```python
from build123d import *

# Parameters (mm, degrees)
SKETCH1_W                = 120
SKETCH1_H                = 120
BOSS_EXTRUDE1_DEPTH      = 115
SHELL1_T                 = -5
BOSS_EXTRUDE2_START      = -5
BOSS_EXTRUDE2_DEPTH      = 10
BOSS_EXTRUDE3_DEPTH      = 5
BOSS_EXTRUDE3_DEPTH_BACK = 5


# Read off the part's stored shape, not the designer's step: Boss-Extrude2
with BuildPart() as part:
    # Sketch1 → Boss-Extrude1 (new body)
    with BuildSketch(Plane(origin=(0, 0, 0), x_dir=(1, 0, 0), z_dir=(0, 1, 0))):
        Rectangle(SKETCH1_W, SKETCH1_H)
    extrude(amount=BOSS_EXTRUDE1_DEPTH)

    # Shell1
    shell1_openings = [part.faces().sort_by_distance(p)[0] for p in [
        (0, 115, 0),
    ]]
    offset(amount=SHELL1_T, openings=shell1_openings, kind=Kind.INTERSECTION)

    # Boss-Extrude2 outline → Boss-Extrude2 (add)
    with BuildSketch(Plane(origin=(0, 0, 0), x_dir=(0.7071067811865475, 0, 0.7071067811865477), z_dir=(-0.7071067811865477, 0, 0.7071067811865475)).offset(BOSS_EXTRUDE2_START)):
        with BuildLine():
            Line((-78.852813742, 20.605551275), (-78.852813742, 25))
            ThreePointArc((-78.852813742, 25), (-79.342915027, 25.345119301), (-79.852813742, 25.660254038))
            ThreePointArc((-79.852813742, 25.660254038), (-94.852813742, 17), (-79.852813742, 8.339745962))
            ThreePointArc((-79.852813742, 8.339745962), (-79.342915027, 8.654880699), (-78.852813742, 9))
            Line((-78.852813742, 9), (-78.852813742, 13.394448725))
            ThreePointArc((-78.852813742, 13.394448725), (-79.314922525, 12.718439436), (-79.852813742, 12.101020514))
            ThreePointArc((-79.852813742, 12.101020514), (-91.852813742, 17), (-79.852813742, 21.898979486))
            ThreePointArc((-79.852813742, 21.898979486), (-79.314922525, 21.281560564), (-78.852813742, 20.605551275))
        make_face()
        with BuildLine():
            Line((-78.852813742, 106.605551275), (-78.852813742, 111))
            ThreePointArc((-78.852813742, 111), (-79.342915027, 111.345119301), (-79.852813742, 111.660254038))
            ThreePointArc((-79.852813742, 111.660254038), (-94.852813742, 103), (-79.852813742, 94.339745962))
            ThreePointArc((-79.852813742, 94.339745962), (-79.342915027, 94.654880699), (-78.852813742, 95))
            Line((-78.852813742, 95), (-78.852813742, 99.394448725))
            ThreePointArc((-78.852813742, 99.394448725), (-79.314922525, 98.718439436), (-79.852813742, 98.101020514))
            ThreePointArc((-79.852813742, 98.101020514), (-91.852813742, 103), (-79.852813742, 107.898979486))
            ThreePointArc((-79.852813742, 107.898979486), (-79.314922525, 107.281560564), (-78.852813742, 106.605551275))
        make_face()
        with BuildLine():
            ThreePointArc((78.852813742, 95), (94.852813742, 103), (78.852813742, 111))
            Line((78.852813742, 111), (78.852813742, 106.605551275))
            ThreePointArc((78.852813742, 106.605551275), (91.852813742, 103), (78.852813742, 99.394448725))
            Line((78.852813742, 99.394448725), (78.852813742, 95))
        make_face()
        with BuildLine():
            ThreePointArc((78.852813742, 9), (94.852813742, 17), (78.852813742, 25))
            Line((78.852813742, 25), (78.852813742, 20.605551275))
            ThreePointArc((78.852813742, 20.605551275), (91.852813742, 17), (78.852813742, 13.394448725))
            Line((78.852813742, 13.394448725), (78.852813742, 9))
        make_face()
    extrude(amount=BOSS_EXTRUDE2_DEPTH)

    # Sketch3 → Boss-Extrude3 (add, two sides: drawn at the far end of the back side and taken through both)
    with BuildSketch(Plane(origin=(0, 0, 0), x_dir=(0.7071067811865475, 0, -0.7071067811865476), z_dir=(0.7071067811865476, 0, 0.7071067811865475)).offset(-BOSS_EXTRUDE3_DEPTH_BACK)):
        with BuildLine():
            Line((-78.852813742, 111), (-78.852813742, 106.605551275))
            ThreePointArc((-78.852813742, 106.605551275), (-91.852813742, 103), (-78.852813742, 99.394448725))
            Line((-78.852813742, 99.394448725), (-78.852813742, 95))
            ThreePointArc((-78.852813742, 95), (-94.852813742, 103), (-78.852813742, 111))
        make_face()
        with BuildLine():
            Line((78.852813742, 111), (78.852813742, 106.605551275))
            ThreePointArc((78.852813742, 106.605551275), (91.852813742, 103), (78.852813742, 99.394448725))
            Line((78.852813742, 99.394448725), (78.852813742, 95))
            ThreePointArc((78.852813742, 95), (94.852813742, 103), (78.852813742, 111))
        make_face()
        with BuildLine():
            Line((-78.852813742, 13.394448725), (-78.852813742, 9))
            ThreePointArc((-78.852813742, 9), (-94.852813742, 17), (-78.852813742, 25))
            Line((-78.852813742, 25), (-78.852813742, 20.605551275))
            ThreePointArc((-78.852813742, 20.605551275), (-91.852813742, 17), (-78.852813742, 13.394448725))
        make_face()
        with BuildLine():
            Line((78.852813742, 25), (78.852813742, 20.605551275))
            ThreePointArc((78.852813742, 20.605551275), (91.852813742, 17), (78.852813742, 13.394448725))
            Line((78.852813742, 13.394448725), (78.852813742, 9))
            ThreePointArc((78.852813742, 9), (94.852813742, 17), (78.852813742, 25))
        make_face()
    extrude(amount=BOSS_EXTRUDE3_DEPTH + BOSS_EXTRUDE3_DEPTH_BACK)


solid = part.part
```
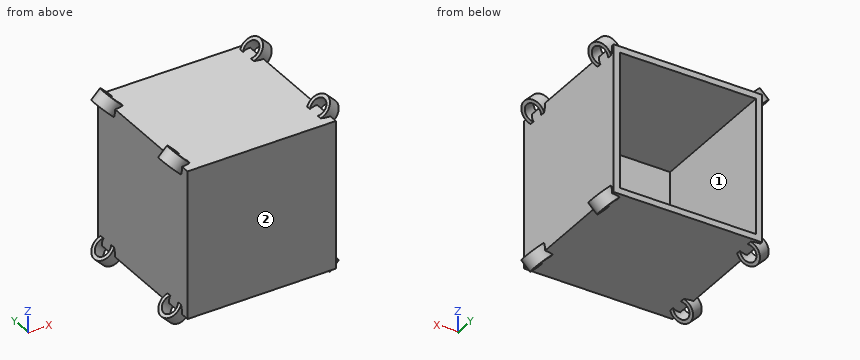
Source: CAD feature listing. Evaluate the final solid. Frame: model axes, mm. Face numbers are marked on the shaded views. Coordinates: 2 decimals unless noted, no trailing zeros. Write each loop counter-clockwise with the first axis right and the second up, starting at its lowest first coordinate (ties: lowest second). Pieces come first, ordered by that corner, then holes. Notation, with made-up numbers: M 64,-32 L 96,-32 A33 cw 96,0 Z; hole C 86.25,11.5 d6. An arc over 180 degrees is marked long. Answer as a JSON object with one key per item and string values.
1. Cut plane D-D on x = -31. Output: boundary loops of the cut face in (y, z), plus the area to 3 significant figures.
Evaluation:
{"outline": "M 0,-60 L 115,-60 L 115,-55 L 5,-55 L 5,55 L 115,55 L 115,60 L 0,60 Z", "area": "1,700 mm^2"}
2. Ray query, L1, parallel to X at y = 20, z = -44.5; L2, parallel to Y at x = -20.5, z = -5. Return the intervals inside material, ascending.
Evaluation:
{"L1": "-60 to -55, 55 to 60", "L2": "0 to 5"}
3. Cut plane A-A on y = 16. Output: boundary loops of the cut face in (x, z).
Evaluation:
{"outline": "M -70.57,-63.5 L -63.5,-70.57 L -61.36,-68.43 L -68.43,-61.36 Z; M -70.57,63.5 L -68.43,61.36 L -61.36,68.43 L -63.5,70.57 Z; M -60,-60 L 60,-60 L 60,60 L -60,60 Z; M 61.36,-68.43 L 63.5,-70.57 L 70.57,-63.5 L 68.43,-61.36 Z; M 61.36,68.43 L 68.43,61.36 L 70.57,63.5 L 63.5,70.57 Z; hole M -55,-55 L 55,-55 L 55,55 L -55,55 Z"}
4. Draft query along Z for the marked faces 1 and 2. Return one class per face: released by +Z, released by -Z, zero draft, split by the parting line, or undercut.
Evaluation:
{"face 1": "undercut", "face 2": "zero draft"}
5. Cut plane B-B on y = 47. Output: boundary loops of the cut face in (x, z).
Evaluation:
{"outline": "M -60,-60 L 60,-60 L 60,60 L -60,60 Z; hole M -55,-55 L 55,-55 L 55,55 L -55,55 Z"}
6. Contact query for flat-ended pins moving along their axis: P1, Ø8, axis at y = 77.5, z = 11, coming from the +X side; P2, Ø8, axis at x = 5, z = -1, coming from the +Y side; P3, Ø1, axis at x = -39.5, y = 69.5, coming from the -Z side. Output: stop coordinate, or through.
Evaluation:
{"P1": "x = 60", "P2": "y = 5", "P3": "z = -60"}
7. Cut plane C-C on z = 26.5. Output: boundary loops of the cut face in (x, y).
Evaluation:
{"outline": "M -60,0 L 60,0 L 60,115 L 55,115 L 55,5 L -55,5 L -55,115 L -60,115 Z"}
